Autodesk Fusion 360 part; units mm, degrees
sketch "Sketch1" plane through (0, 0, 0) normal (0, 1, 0) x (1, 0, 0)
  line L0 (15, -15) -> (-15, -15)
  line L1 (-15, -15) -> (-15, 15)
  line L2 (-15, 15) -> (15, 15)
  line L3 (15, 15) -> (15, -15)
  line L4 (15, -15) -> (-15, 15) construction
  line L5 (-15, -15) -> (15, 15) construction
  line L6 (-4.05, -15) -> (-4.05, -12.8)
  line L7 (-4.05, -12.8) -> (-11.2444, -12.8)
  line L8 (-11.2444, -12.8) -> (-4.3444, -5.9)
  line L9 (-4.3444, -5.9) -> (0, -5.9)
  line L10 (0, 0) -> (0, -15) construction
  line L11 (4.05, -15) -> (4.05, -12.8)
  line L12 (4.05, -12.8) -> (11.2444, -12.8)
  line L13 (11.2444, -12.8) -> (4.3444, -5.9)
  line L14 (4.3444, -5.9) -> (0, -5.9)
  dimension "d1" = 30
  dimension "d2" = 30
  dimension "d3" = 8.1
  dimension "d4" = 9.1
  dimension "d6" = 2.2
  dimension "d7" = 1.1
sketch "Sketch2" plane through (0, 0, 0) normal (0, 1, 0) x (1, 0, 0)
  line L0 (15, -15) -> (-15, -15) construction
  line L1 (3.5, -15) -> (3.5, -12.9)
  line L2 (3.5, -12.9) -> (8.5, -12.9)
  line L3 (8.5, -12.9) -> (4.5, -8.9)
  line L4 (3.5, -15) -> (12, -15)
  line L5 (12, -15) -> (12, -16.35)
  line L6 (12, -16.35) -> (-8.15, -16.35)
  arc A0 (-8.15, -16.35) -> (-8.15, -21.35) centre (-8.15, -18.85) ccw
  line L7 (-8.15, -21.35) -> (8, -21.35)
  line L8 (8, -21.35) -> (8, -17.75)
  line L9 (9.7071, -17.0429) -> (12, -19.3358)
  line L10 (12, -19.3358) -> (12, -22.7)
  line L11 (12, -22.7) -> (-8.15, -22.7)
  arc A1 (-8.15, -15) -> (-8.15, -22.7) centre (-8.15, -18.85) ccw
  line L12 (-8.15, -15) -> (-3.5, -15)
  line L13 (-3.5, -15) -> (-3.5, -12.9)
  line L14 (-3.5, -12.9) -> (-8.5, -12.9)
  line L15 (-11.2444, -12.8) -> (-4.3444, -5.9) construction
  line L16 (-8.5, -12.9) -> (-4.5, -8.9)
  line L17 (-4.5, -8.9) -> (4.5, -8.9)
  line L18 (-12, -18.85) -> (-12, -26.3495) construction
  line L19 (-15, -15) -> (-15, 15)
  line L20 (15, 15) -> (15, -15)
  line L21 (0, 0) -> (0, -24.1039) construction
  arc A2 (9.7071, -17.0429) -> (8, -17.75) centre (9, -17.75) ccw
  point P0 (8, -15.3358)
  dimension "d8" = 3
  dimension "d9" = 3
  dimension "d12" = 1.35
  dimension "d13" = 4
  dimension "d14" = 7
  dimension "d15" = 17
  dimension "d18" = 4
  dimension "d19" = 5
  dimension "d20" = 45
  dimension "d25" = 1
  dimension "d26" = 1.4
  dimension "d40" = 2.1
extrude "Extrude1" add sketch "Sketch2" along normal mid plane 7
chamfer "Chamfer1" distance 2 angle 45 4 edges at (-3.5, -3.5, 13.95) (3.5, -3.5, 13.95) (3.5, 3.5, 13.95) (-3.5, 3.5, 13.95)
sketch "Sketch3" plane through (0, 0, 0) normal (0, 0, 1) x (1, 0, 0)
  circle A0 centre (0, 0) radius 4
  circle A1 centre (0, 0) radius 8.25
  dimension "d24" = 8
  dimension "d29" = 16.5
fillet "Fillet1" radius 2.5 2 edges at (8, 0, 21.35) (12, 0, 22.7)
fillet "Fillet2" radius 1 4 edges at (8.5, 0, 12.9) (4.5, 0, 8.9) (-4.5, 0, 8.9) (-8.5, 0, 12.9)
sketch "Sketch4" plane through (0, 0, 0) normal (0, 1, 0) x (1, 0, 0)
  line L0 (-1.5, -15) -> (-8.15, -15)
  line L1 (-6.325, -15) -> (-6.325, -14.9)
  arc A0 (-4.825, -15) -> (-6.325, -14.9) centre (-6.325, -26.2) ccw
  line L2 (-6.325, -14.9) -> (-5.7947, -14.9) construction
  dimension "d30" = 0.1
  dimension "d31" = 1.5
equation "d12 = ( 0.45 * 3 ) * 1 mm"
Model file for the job. Use its own axes, mm. A direction names the side the tool comes from. Give positions to 0.01 mm unless a question says otherwise; leave off trailing zeros. Loops run counter-clockwise (first coordinate to the right, second up) from the corner with the lowest first, then second, coordinate; pieces in that order, holes last.
Item 1: Drill centre lines: line 1 along Z through (x, y) = (-2.75, 3); line 2 along Z through (x, y) = (-8.25, 2); line 3 along Z through (x, y) = (1.75, 3). Where is each one in solid material? Low to high.
Check values:
line 1: z = 8.9 to 12.9, 15 to 16.35, 21.35 to 22.7
line 2: z = 15 to 16.35, 21.35 to 22.7
line 3: z = 8.9 to 16.35, 21.35 to 22.7
Item 2: Slice it at C-C (x = -4.5). Write the cut outline in (y, z).
Check values:
outline: (-3.5, 8.99) - (3.5, 8.99) - (3.5, 12.9) - (-3.5, 12.9) - close; (-3.5, 15) - (3.5, 15) - (3.5, 16.35) - (-3.5, 16.35) - close; (-3.5, 21.35) - (3.5, 21.35) - (3.5, 22.7) - (-3.5, 22.7) - close
Item 3: Drop flat-ended pins along their axis: P1, Ø3, axis at y = 1.5, z = 11.5, coming from the +X side; P2, Ø1.5, axis at x = -8, z = 20.5, coming from the +Y side; P3, Ø1.7, axis at y = -0.5, z = 14, coming from the -X side; P4, Ø0.6, axis at y = 0.5, z = 18, coming from the -X side. Give the stop position or say it passes through.
Check values:
P1: stops at x = 7.09
P2: passes through
P3: stops at x = -3.5
P4: stops at x = -11.96
Item 4: Slice it at A-A (z = 14.5). Write the cut outline in (x, y).
Check values:
outline: (-3.5, -1.5) - (-1.5, -3.5) - (1.5, -3.5) - (3.5, -1.5) - (3.5, 1.5) - (1.5, 3.5) - (-1.5, 3.5) - (-3.5, 1.5) - close
Item 5: Which spindle directions (+Z, -Z, +X, -X, +Y, -Y) get a long thin tool onto all of the face, cutting with end or side? Do faces 5 (the face through (2, 0, 16.35)), 6 (the face through (2, -3, 14)), 7 (the face through (8, 0, 18)). Say none if no direction does.
Check values:
face 5: +X, +Y, -Y
face 6: +X, -Y
face 7: +Y, -Y
Item 6: Mould opens along Z. For faces 1 (the face through (-12, 0, 18.9)), 2 (the face through (-5.8, 0, 10.2)), 3 (the face through (11.287, -0.049, 21.948)), 4 (the face through (-10.65, -0.05, 18.9)) say: +Z half, -Z half, draft (parallel to the pull), parting line (faces both ways), or undercut.
Check values:
face 1: parting line
face 2: -Z half
face 3: +Z half
face 4: undercut
Item 7: Slice it at D-D (y = -3). Write the cut outline in (x, z).
Check values:
outline: (-8.15, 15) - (-2, 15) - (-2, 12.9) - (-6.09, 12.9) arc R1 ccw to (-6.79, 11.19) - (-4.79, 9.19) arc R1 ccw to (-4.09, 8.9) - (4.09, 8.9) arc R1 ccw to (4.79, 9.19) - (6.79, 11.19) arc R1 ccw to (6.09, 12.9) - (2, 12.9) - (2, 15) - (12, 15) - (12, 16.35) - (-8.15, 16.35) arc R2.5 cw to (-8.15, 21.35) - (5.5, 21.35) arc R2.5 cw to (8, 18.85) - (8, 17.75) arc R1 ccw to (9.71, 17.04) - (12, 19.34) - (12, 20.2) arc R2.5 ccw to (9.5, 22.7) - (-8.15, 22.7) arc R3.85 ccw to start
Item 8: Slice it at B-B (y = -2). Write the cut outline in (x, z), plus the area to 3 significant figures.
Check values:
outline: (-8.15, 15) - (-3, 15) - (-3, 12.9) - (-6.09, 12.9) arc R1 ccw to (-6.79, 11.19) - (-4.79, 9.19) arc R1 ccw to (-4.09, 8.9) - (4.09, 8.9) arc R1 ccw to (4.79, 9.19) - (6.79, 11.19) arc R1 ccw to (6.09, 12.9) - (3, 12.9) - (3, 15) - (12, 15) - (12, 16.35) - (-8.15, 16.35) arc R2.5 cw to (-8.15, 21.35) - (5.5, 21.35) arc R2.5 cw to (8, 18.85) - (8, 17.75) arc R1 ccw to (9.71, 17.04) - (12, 19.34) - (12, 20.2) arc R2.5 ccw to (9.5, 22.7) - (-8.15, 22.7) arc R3.85 ccw to start
area: 145 mm2
